Could you check a few things on this drawing? It's one solid part, dimensions in mm from its lowest x, y, z. A direction names the side the tool comes from. Give positions to 0.01 mm unless a question says otherwise; leave off trailing zeros. Loops run counter-clockwise (first coordinate to the right, second up) from the corner with the lowest first, then second, coordinate; pieces in that order, holes last. Notation, with made-up numbers: M 60,24.5 L 86,24.5 A28 cw 86,42.5 Z; hole C 14.5,75 d7. An arc over 180 degrees is marked long. Answer in a Markdown table with one row per item. Add a question column.
1. If we section it at D-D on y = 16.5: List the corners of the cut face in (x, z) for me.
2. If we section it at B-B on y = 41: List the corners of the cut face in (x, z) for me, then the cut area to 3 significant figures.
3. If we section it at A-A on z = 50: List the corners of the cut face in (x, y) for me, then the cut area to 3 significant figures.
4. If we section it at C-C on x = 141: List the corners of the cut face in (y, z) for me.
5. I need wall thicknesses on line 1 along Y through (x, z) = (11.5, 52.5); line 2 along X through (y, z) = (18, 21); line 3 along X through (y, z) = (29.5, 8.5). Which ranges of each line are inside material? Lowest first, please. Write a range as from..to.
6. Thinking about a two-plate mould opening in X: for the marked faces 4, 5 and 6, which applies, released by +X, released by -X, zero draft, split by the parting line, or undercut?
7. I'm going to push flat-ended pins straight in: pin 1 Ø19 at (x, z) = (130.5, 41) entering from +Y; pin 2 Ø8 at (y, z) = (45.5, 24) entering from +X; pin 3 Ø19 at (y, z) = (30.5, 16) entering from -X. Where does each tip first touch, or does it pass through?
8. Which directions (+Z, -Z, +X, -X, +Y, -Y) give clear straight access to the entire face, cutting with the end or side of a thin tool? Please do the marked faces 1, 2 and 3.
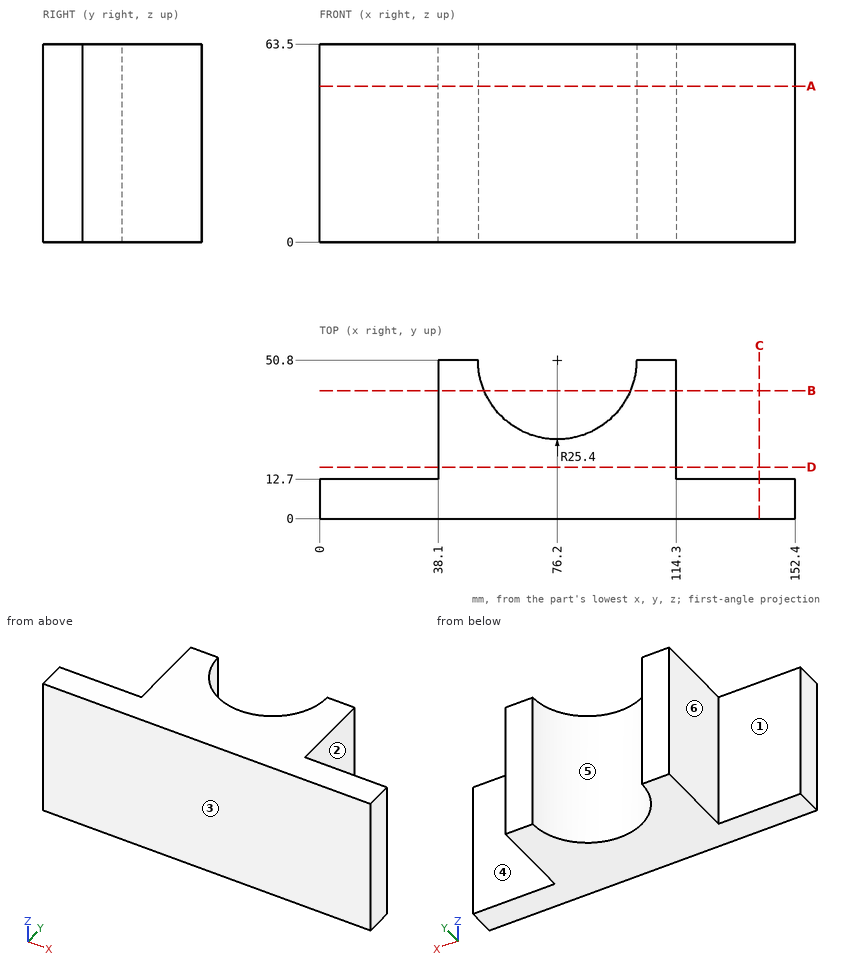
Results:
| question | item | result |
|---|---|---|
| 1 | outline | M 38.1,0 L 114.3,0 L 114.3,63.5 L 38.1,63.5 Z |
| 2 | outline | M 38.1,0 L 52.77,0 L 52.77,63.5 L 38.1,63.5 Z; M 99.63,0 L 114.3,0 L 114.3,63.5 L 99.63,63.5 Z |
| 2 | area | 1,860 mm2 |
| 3 | outline | M 0,0 L 152.4,0 L 152.4,12.7 L 114.3,12.7 L 114.3,50.8 L 101.6,50.8 A25.4 cw 50.8,50.8 L 38.1,50.8 L 38.1,12.7 L 0,12.7 Z |
| 3 | area | 3,830 mm2 |
| 4 | outline | M 0,0 L 12.7,0 L 12.7,63.5 L 0,63.5 Z |
| 5 | line 1 | 0..12.7 |
| 5 | line 2 | 38.1..114.3 |
| 5 | line 3 | 38.1..62.36, 90.04..114.3 |
| 6 | face 4 | zero draft |
| 6 | face 5 | undercut |
| 6 | face 6 | released by -X |
| 7 | pin 1 | y = 12.7 |
| 7 | pin 2 | x = 114.3 |
| 7 | pin 3 | x = 38.1 |
| 8 | face 1 | +Z, -Z, -X, +Y |
| 8 | face 2 | +Z, -Z, +X, +Y |
| 8 | face 3 | +Z, -Z, +X, -X, -Y |
